Can you work these out from the model? Positions are in its coordinate system, mm. A direction names the side the tool comes from. Give positions to 0.01 mm unless a question says otherwise; leave off trailing zeros. Loops run counter-clockwise (first coordinate to the right, second up) from the corner with the lowest first, then second, coordinate; pieces in that order, holes last.
from build123d import *

# Parameters (mm, degrees)
F0_R     = 10
F0_R_2   = 1.5
F1_DEPTH = 9


# Not quite as in the source:
# - a feature names something its author has since deleted; it is built from what else it names


with BuildPart() as f1:
    # F0 (on Top) → F1 (new body)
    with BuildSketch(Plane.XY):
        Circle(F0_R)
        with BuildLine():
            Line((-3.2035890311, -6.37527581), (-1.8173406245, -3.6165836534))
            ThreePointArc((-1.8173406245, -3.6165836534), (0.5722008428, -4.0068679119), (2.756987683, -2.9633466189))
            Line((2.756987683, -2.9633466189), (4.8599890306, -5.2237564028))
            ThreePointArc((4.8599890306, -5.2237564028), (1.0086696565, -7.0632648157), (-3.2035890311, -6.37527581))
        make_face(mode=Mode.SUBTRACT)
        with BuildLine():
            ThreePointArc((-4.8599890306, 5.2237564028), (-1.0086696565, 7.0632648157), (3.2035890311, 6.37527581))
            Line((3.2035890311, 6.37527581), (1.8173406245, 3.6165836534))
            ThreePointArc((1.8173406245, 3.6165836534), (-0.5722008428, 4.0068679119), (-2.756987683, 2.9633466189))
            Line((-2.756987683, 2.9633466189), (-4.8599890306, 5.2237564028))
        make_face(mode=Mode.SUBTRACT)
        Circle(F0_R_2, mode=Mode.SUBTRACT)
    extrude(amount=F1_DEPTH)


solid = f1.part
(1) Suppose I cut it at C-C on z = 8.5. List the corners of the cut face in (x, y) for me.
Returned:
outline: circle Ø20 at (0, 0); hole (-4.86, 5.22) - (-2.76, 2.96) arc R4.05 cw to (1.82, 3.62) - (3.2, 6.38) arc R7.13 ccw to start; hole (-3.2, -6.38) arc R7.13 ccw to (4.86, -5.22) - (2.76, -2.96) arc R4.05 cw to (-1.82, -3.62) - close; hole circle Ø3 at (0, 0)
(2) Suppose I cut it at B-B on y = 0. List the corners of the cut face in (x, z) for me, plus the area to 3 significant figures.
Returned:
outline: (-10, 0) - (-1.5, 0) - (-1.5, 9) - (-10, 9) - close; (1.5, 0) - (10, 0) - (10, 9) - (1.5, 9) - close
area: 153 mm2
(3) Which directions (+Z, -Z, +X, -X, +Y, -Y) give clear straight access to the entire face, cutting with the end or side of a thin tool? Please do faces 1 (the cylindrical face through (1.069, -7.054, 4.437)), 2 (the flat face through (0, -2, 0)).
Returned:
face 1: +Z, -Z
face 2: -Z, +X, -X, +Y, -Y
(4) Suppose I cut it at A-A on x = 0. List the corners of the cut face in (y, z) for me, plus the area to 3 significant figures.
Returned:
outline: (-10, 0) - (-7.13, 0) - (-7.13, 9) - (-10, 9) - close; (-4.05, 0) - (-1.5, 0) - (-1.5, 9) - (-4.05, 9) - close; (1.5, 0) - (4.05, 0) - (4.05, 9) - (1.5, 9) - close; (7.13, 0) - (10, 0) - (10, 9) - (7.13, 9) - close
area: 97.4 mm2
(5) Thinking about a two-plate mould opening in X: for faces 3 (the cylindrical face through (0.54, -4.01, 4.44)), 4 (the cylindrical face through (-2.17, -9.76, 4.44)), 5 (the flat face through (0, -2, 9)), which applies, pulls with the +X half, pulls with the -X half, needs draft (parallel to the pull), parting line crosses it, or undercut?
Returned:
face 3: undercut
face 4: parting line crosses it
face 5: needs draft
(6) Suppose I cut it at D-D on x = 2.25. List the corners of the cut face in (y, z) for me.
Returned:
outline: (-9.74, 0) - (-6.77, 0) - (-6.77, 9) - (-9.74, 9) - close; (-3.36, 0) - (4.48, 0) - (4.48, 9) - (-3.36, 9) - close; (6.77, 0) - (9.74, 0) - (9.74, 9) - (6.77, 9) - close
(7) Will this pin go through, and if not, where does the flat tip stop? P1, Ø1.5, axis at x = -1, z = 4, coming from the -Y side.
Returned:
P1: stops at y = -10
(8) Please list where these lines run through material, in increasing order: probe 1 along Y at (x, z) = (0, 5); probe 2 along Y at (x, z) = (-7, 4.5); probe 3 along X at (y, z) = (6, 3).
Returned:
probe 1: y = -10 to -7.13, -4.05 to -1.5, 1.5 to 4.05, 7.13 to 10
probe 2: y = -7.14 to 7.14
probe 3: x = -8 to -3.86, 3.02 to 8
